```python
from build123d import *

# Parameters (mm, degrees)
BOSS_EXTRUDE1_DEPTH = 4
CUT_EXTRUDE1_REACH  = 123.301
SKETCH6_R           = 1.5
SKETCH6_R_2         = 2.5
SKETCH6_W           = 20
SKETCH6_H           = 40
SKETCH7_R           = 1.5
CUT_EXTRUDE2_DEPTH  = 122.300839153
SKETCH8_W           = 5.5
SKETCH8_H           = 10
CUT_EXTRUDE3_DEPTH  = 122.300839153
SKETCH9_R           = 1.5
SKETCH9_R_2         = 14
CUT_EXTRUDE4_DEPTH  = 122.300839153


with BuildPart() as part:
    # Sketch1 → Boss-Extrude1 (new body)
    with BuildSketch(Plane(origin=(0, 0, 0), x_dir=(1, 0, 0), z_dir=(0, 1, 0))):
        with BuildLine():
            Line((0, -78.772581113), (0, 81.227418887))
            Line((0, 81.227418887), (67.544155877, 81.227418887))
            ThreePointArc((67.544155877, 81.227418887), (68.692206174, 80.999057485), (69.665476221, 80.348739231))
            Line((69.665476221, 80.348739231), (89.121320344, 60.892895108))
            ThreePointArc((89.121320344, 60.892895108), (89.771638598, 59.919625062), (90, 58.771574765))
            Line((90, 58.771574765), (90, -56.31673699))
            ThreePointArc((90, -56.31673699), (89.771638598, -57.464787287), (89.121320344, -58.438057333))
            Line((89.121320344, -58.438057333), (69.665476221, -77.893901456))
            ThreePointArc((69.665476221, -77.893901456), (68.692206174, -78.54421971), (67.544155877, -78.772581113))
            Line((67.544155877, -78.772581113), (0, -78.772581113))
        make_face()
    boss_extrude1 = extrude(amount=BOSS_EXTRUDE1_DEPTH)

    # Sketch6 → Cut-Extrude1 (cut, up to next)
    with BuildSketch(Plane(origin=(0, 4, 0), x_dir=(1, 0, 0), z_dir=(0, 1, 0)), mode=Mode.PRIVATE) as cut_extrude1_sk1:
        with Locations(Location((67.009618943, 32.627418887, 0), (0, 0, 270))):
            Circle(SKETCH6_R)
    cut_extrude1_tool1 = extrude(cut_extrude1_sk1.sketch, amount=-CUT_EXTRUDE1_REACH, mode=Mode.PRIVATE) & part.part
    # Sketch6 → Cut-Extrude1 (cut, up to next)
    with BuildSketch(Plane(origin=(0, 4, 0), x_dir=(1, 0, 0), z_dir=(0, 1, 0)), mode=Mode.PRIVATE) as cut_extrude1_sk2:
        with Locations(Location((77.009618943, 32.627418887, 0), (0, 0, 270))):
            Circle(SKETCH6_R)
    cut_extrude1_tool2 = extrude(cut_extrude1_sk2.sketch, amount=-CUT_EXTRUDE1_REACH, mode=Mode.PRIVATE) & part.part
    # Sketch6 → Cut-Extrude1 (cut, up to next)
    with BuildSketch(Plane(origin=(0, 4, 0), x_dir=(1, 0, 0), z_dir=(0, 1, 0)), mode=Mode.PRIVATE) as cut_extrude1_sk3:
        with Locations(Location((77.009618943, -15.172581113, 0), (0, 0, 270))):
            Circle(SKETCH6_R)
    cut_extrude1_tool3 = extrude(cut_extrude1_sk3.sketch, amount=-CUT_EXTRUDE1_REACH, mode=Mode.PRIVATE) & part.part
    # Sketch6 → Cut-Extrude1 (cut, up to next)
    with BuildSketch(Plane(origin=(0, 4, 0), x_dir=(1, 0, 0), z_dir=(0, 1, 0)), mode=Mode.PRIVATE) as cut_extrude1_sk4:
        with Locations(Location((67.009618943, -15.172581113, 0), (0, 0, 270))):
            Circle(SKETCH6_R)
    cut_extrude1_tool4 = extrude(cut_extrude1_sk4.sketch, amount=-CUT_EXTRUDE1_REACH, mode=Mode.PRIVATE) & part.part
    # Sketch6 → Cut-Extrude1 (cut, up to next)
    with BuildSketch(Plane(origin=(0, 4, 0), x_dir=(1, 0, 0), z_dir=(0, 1, 0)), mode=Mode.PRIVATE) as cut_extrude1_sk5:
        with Locations(Location((72.009618943, 53.727418887, 0), (0, 0, 270))):
            Circle(SKETCH6_R_2)
    cut_extrude1_tool5 = extrude(cut_extrude1_sk5.sketch, amount=-CUT_EXTRUDE1_REACH, mode=Mode.PRIVATE) & part.part
    # Sketch6 → Cut-Extrude1 (cut, up to next)
    with BuildSketch(Plane(origin=(0, 4, 0), x_dir=(1, 0, 0), z_dir=(0, 1, 0)), mode=Mode.PRIVATE) as cut_extrude1_sk6:
        with Locations(Location((72.009618943, -51.272581113, 0), (0, 0, 270))):
            Circle(SKETCH6_R_2)
    cut_extrude1_tool6 = extrude(cut_extrude1_sk6.sketch, amount=-CUT_EXTRUDE1_REACH, mode=Mode.PRIVATE) & part.part
    # Sketch6 → Cut-Extrude1 (cut, up to next)
    with BuildSketch(Plane(origin=(0, 4, 0), x_dir=(1, 0, 0), z_dir=(0, 1, 0)), mode=Mode.PRIVATE) as cut_extrude1_sk7:
        with Locations((72.009618943, 8.727418887)):
            Rectangle(SKETCH6_W, SKETCH6_H)
    cut_extrude1_tool7 = extrude(cut_extrude1_sk7.sketch, amount=-CUT_EXTRUDE1_REACH, mode=Mode.PRIVATE) & part.part
    cut_extrude1_1 = cut_extrude1_tool1.solids().sort_by_distance((67.009619, 4, -32.627419))[0]
    add(cut_extrude1_1, mode=Mode.SUBTRACT)
    cut_extrude1_2 = cut_extrude1_tool2.solids().sort_by_distance((77.009619, 4, -32.627419))[0]
    add(cut_extrude1_2, mode=Mode.SUBTRACT)
    cut_extrude1_3 = cut_extrude1_tool3.solids().sort_by_distance((77.009619, 4, 15.172581))[0]
    add(cut_extrude1_3, mode=Mode.SUBTRACT)
    cut_extrude1_4 = cut_extrude1_tool4.solids().sort_by_distance((67.009619, 4, 15.172581))[0]
    add(cut_extrude1_4, mode=Mode.SUBTRACT)
    cut_extrude1_5 = cut_extrude1_tool5.solids().sort_by_distance((72.009619, 4, -53.727419))[0]
    add(cut_extrude1_5, mode=Mode.SUBTRACT)
    cut_extrude1_6 = cut_extrude1_tool6.solids().sort_by_distance((72.009619, 4, 51.272581))[0]
    add(cut_extrude1_6, mode=Mode.SUBTRACT)
    cut_extrude1_7 = cut_extrude1_tool7.solids().sort_by_distance((72.009619, 4, -8.727419))[0]
    add(cut_extrude1_7, mode=Mode.SUBTRACT)
    cut_extrude1 = cut_extrude1_1 + cut_extrude1_2 + cut_extrude1_3 + cut_extrude1_4 + cut_extrude1_5 + cut_extrude1_6 + cut_extrude1_7  # Cut-Extrude1 as one shape, for the pattern or mirror that repeats it

    # Sketch7 → Cut-Extrude2 (cut, through all)
    with BuildSketch(Plane(origin=(0, 4, 0), x_dir=(1, 0, 0), z_dir=(0, 1, 0))):
        with BuildLine():
            Line((11, -51.772581113), (0, -51.772581113))
            Line((0, -51.772581113), (0, -54.772581113))
            Line((0, -54.772581113), (11, -54.772581113))
            ThreePointArc((11, -54.772581113), (11.925367624, -53.272581113), (11, -51.772581113))
        make_face()
        with BuildLine():
            Line((0, -19.772581113), (0, -22.772581113))
            Line((0, -22.772581113), (11, -22.772581113))
            ThreePointArc((11, -22.772581113), (12.5, -21.272581113), (11, -19.772581113))
            Line((11, -19.772581113), (0, -19.772581113))
        make_face()
        with BuildLine():
            Line((57.544155877, -60.772581113), (0, -60.772581113))
            Line((0, -60.772581113), (0, -78.772581113))
            Line((0, -78.772581113), (62.544155877, -78.772581113))
            ThreePointArc((62.544155877, -78.772581113), (60.422835534, -77.893901456), (59.544155877, -75.772581113))
            Line((59.544155877, -75.772581113), (59.544155877, -62.772581113))
            ThreePointArc((59.544155877, -62.772581113), (58.95836944, -61.35836755), (57.544155877, -60.772581113))
        make_face()
        with BuildLine():
            Line((0, 81.227418887), (0, 76.227418887))
            Line((0, 76.227418887), (46.431936457, 76.227418887))
            ThreePointArc((46.431936457, 76.227418887), (48.258220744, 76.847358867), (49.329713936, 78.450961752))
            Line((49.329713936, 78.450961752), (49.477866868, 79.003876023))
            ThreePointArc((49.477866868, 79.003876023), (50.54936006, 80.607478908), (52.375644347, 81.227418887))
            Line((52.375644347, 81.227418887), (0, 81.227418887))
        make_face()
        with BuildLine():
            Line((74.509618943, 45.727418887), (69.509618943, 45.727418887))
            ThreePointArc((69.509618943, 45.727418887), (67.509618943, 43.727418887), (69.509618943, 41.727418887))
            Line((69.509618943, 41.727418887), (74.509618943, 41.727418887))
            ThreePointArc((74.509618943, 41.727418887), (76.509618943, 43.727418887), (74.509618943, 45.727418887))
        make_face()
        with Locations(Location((38, 30.227418887, 0), (0, 0, 270))):
            Circle(SKETCH7_R)
        with Locations(Location((38, -10.772581113, 0), (0, 0, 270))):
            Circle(SKETCH7_R)
    cut_extrude2 = extrude(amount=-CUT_EXTRUDE2_DEPTH, mode=Mode.SUBTRACT)

    # Mirror1: Boss-Extrude1, Cut-Extrude1, Cut-Extrude2 across plane
    add(boss_extrude1.mirror(Plane(origin=(0, 4, 78.772581113), x_dir=(0, 0, 1), z_dir=(1, 0, 0))))
    add(cut_extrude1.mirror(Plane(origin=(0, 4, 78.772581113), x_dir=(0, 0, 1), z_dir=(1, 0, 0))), mode=Mode.SUBTRACT)
    add(cut_extrude2.mirror(Plane(origin=(0, 4, 78.772581113), x_dir=(0, 0, 1), z_dir=(1, 0, 0))), mode=Mode.SUBTRACT)

    # Sketch8 → Cut-Extrude3 (cut, through all)
    with BuildSketch(Plane(origin=(0, 4, 0), x_dir=(1, 0, 0), z_dir=(0, 1, 0))):
        with Locations((-38.25, 22.727418887)):
            Rectangle(SKETCH8_W, SKETCH8_H)
        with BuildLine():
            Line((90, -25.272581113), (90, -39.272581113))
            ThreePointArc((90, -39.272581113), (89.267766953, -37.50481416), (87.5, -36.772581113))
            Line((87.5, -36.772581113), (84.174158586, -36.772581113))
            ThreePointArc((84.174158586, -36.772581113), (82.533118782, -37.386583137), (81.698160388, -38.926990423))
            ThreePointArc((81.698160388, -38.926990423), (76.681626099, -42.995196185), (72.27562777, -38.272581113))
            Line((72.27562777, -38.272581113), (72.27562777, -26.272581113))
            ThreePointArc((72.27562777, -26.272581113), (76.681626099, -21.549966041), (81.698160388, -25.618171802))
            ThreePointArc((81.698160388, -25.618171802), (82.533118782, -27.158579088), (84.174158586, -27.772581113))
            Line((84.174158586, -27.772581113), (87.5, -27.772581113))
            ThreePointArc((87.5, -27.772581113), (89.267766953, -27.040348066), (90, -25.272581113))
        make_face()
    extrude(amount=-CUT_EXTRUDE3_DEPTH, mode=Mode.SUBTRACT)

    # Sketch9 → Cut-Extrude4 (cut, through all)
    with BuildSketch(Plane(origin=(0, 4, 0), x_dir=(1, 0, 0), z_dir=(0, 1, 0))):
        with Locations(Location((-2.69, 30.227418887, 0), (0, 0, 270))):
            Circle(SKETCH9_R)
        with Locations(Location((-38, -33.572581113, 0), (0, 0, 270))):
            Circle(SKETCH9_R)
        with Locations(Location((-2.06, 9.727418887, 0), (0, 0, 270))):
            Circle(SKETCH9_R_2)
    extrude(amount=-CUT_EXTRUDE4_DEPTH, mode=Mode.SUBTRACT)


solid = part.part
```
Verification items for the finished model (mm, model axes). A direction names the side the tool comes from. Give positions to 0.01 mm unless a question says otherwise; leave off trailing zeros. Order: outer loops, then holes, each group sorted by start corner. A loop starts at its lowest first (then second) coordinate and runs counter-clockwise, first axis right, second up. Notation, with made-up numbers: (50, 25.5) -> (102, 25.5) arc R8 ccw to (102, 30.5) -> close; hole circle Ø4 at (11.5, 83). An arc over 180 degrees is marked (long way). Use a Markdown table: item, result.
1) Tool access check on faces 4 (the flat face through (79.257, 1.972, -70.757)), 5 (the cylindrical face through (67.51, 2.03, -43.77)). Record the directions out of +Z, -Z, +X, -X, +Y, -Y that give a thin tool (end or side, any length) a straight path to the whole face; none if there is none.
Results:
| item | result |
|---|---|
| face 4 | -Z, +X, +Y, -Y |
| face 5 | +Y, -Y |
2) Section check C-C, the plane y = 1.15. Give the number of separate pieces and of enclosed holes in the cut face, then the cut area to 3 significant figures.
Results:
| item | result |
|---|---|
| separate pieces | 1 |
| enclosed holes | 26 |
| area | 22,300 mm² |
3) Mould release check, pull along X, two halves, no side actions. Record for faces 1 (the flat face through (90, 2, -17)), 2 (the flat face through (-21, 0, -2)), 3 (the flat face through (72, 2, -28.727)): pulls with the +X half, pulls with the -X half, needs draft (parallel to the pull), parting line crosses it, or undercut.
Results:
| item | result |
|---|---|
| face 1 | pulls with the +X half |
| face 2 | needs draft |
| face 3 | undercut |
4) Material ranges on probe 1 along Z at (x, y) = (37.5, 0.3); probe 2 along Z at (x, y) = (-63, 1.95); probe 3 along X at (y, z) = (1.15, -31), recorded low to high.
Results:
| item | result |
|---|---|
| probe 1 | -76.23 to -31.64, -28.81 to 9.36, 12.19 to 60.77 |
| probe 2 | -81.23 to -28.73, 11.27 to 78.77 |
| probe 3 | -90 to -39.29, -36.71 to -3.98, -1.4 to 36.71, 39.29 to 90 |
5) Section check D-D, the plane x = 17.5. Record the boundary of the cut face in (y, z), then the cut area to 3 significant figures.
Results:
| item | result |
|---|---|
| outline | (0, -76.23) -> (4, -76.23) -> (4, 60.77) -> (0, 60.77) -> close |
| area | 548 mm² |
6) Section check B-B, the plane x = -7. Record the boundary of the cut face in (y, z), then the cut area to 3 significant figures.
Results:
| item | result |
|---|---|
| outline | (0, -76.23) -> (4, -76.23) -> (4, -22.83) -> (0, -22.83) -> close; (0, 3.37) -> (4, 3.37) -> (4, 19.77) -> (0, 19.77) -> close; (0, 22.77) -> (4, 22.77) -> (4, 51.77) -> (0, 51.77) -> close; (0, 54.77) -> (4, 54.77) -> (4, 60.77) -> (0, 60.77) -> close |
| area | 419 mm² |
7) Depth check by flat-ended pin: pin 1 Ø1.7 at (x, y) = (86, 2) entering from +Z; pin 2 Ø1.2 at (x, y) = (-71.5, 2) entering from -Z; pin 3 Ø1.2 at (x, y) = (2, 3) entering from +Z. Enter the tip coordinate at first touch or a pass-through.
Results:
| item | result |
|---|---|
| pin 1 | z = 62.41 |
| pin 2 | z = -79.11 |
| pin 3 | z = 60.77 |
8) Section check A-A, the plane z = -10. Record the boundary of the cut face in (x, y), then the cut area to 3 significant figures.
Results:
| item | result |
|---|---|
| outline | (-90, 0) -> (-82.01, 0) -> (-82.01, 4) -> (-90, 4) -> close; (-62.01, 0) -> (-16.06, 0) -> (-16.06, 4) -> (-62.01, 4) -> close; (11.94, 0) -> (62.01, 0) -> (62.01, 4) -> (11.94, 4) -> close; (82.01, 0) -> (90, 0) -> (90, 4) -> (82.01, 4) -> close |
| area | 448 mm² |
